```python
from build123d import *

# Parameters (mm, degrees)
SALIENTE_EXTRUIR1_DEPTH = 12.7
CORTAR_EXTRUIR20_DEPTH  = 62
CROQUIS12_R             = 26
CROQUIS12_R_2           = 17
CORTAR_EXTRUIR21_DEPTH  = 4
CROQUIS6_R              = 1.25
CORTAR_EXTRUIR22_DEPTH  = 29
CROQUIS13_R             = 1.5
CORTAR_EXTRUIR23_DEPTH  = 29
CROQUIS8_R              = 3
CORTAR_EXTRUIR27_DEPTH  = 64
CROQUIS5_R              = 36
CORTAR_EXTRUIR28_DEPTH  = 4
CROQUIS22_R             = 27
CORTAR_EXTRUIR32_DEPTH  = 1
CORTAR_EXTRUIR33_START  = -1
CROQUIS23_R             = 17
CORTAR_EXTRUIR33_DEPTH  = 1
CROQUIS24_R             = 9
CORTAR_EXTRUIR34_DEPTH  = 67


with BuildPart() as part:
    # Croquis2 → Saliente-Extruir1 (new body)
    with BuildSketch(Plane.XY):
        with BuildLine():
            add(Edge.make_bspline(
                [(318.003849686, 21.000507192), (228.612845689, 50.579171404), (93.837740705, 69.713331037), (-40.897656903, 33.469788637), (-68.237071347, 4.559111896)],
                knots=[0, 0, 0, 0, 0.7074371, 1, 1, 1, 1], degree=3))
            Line((-68.237071347, 4.559111896), (-59.653213383, -5.20395025))
            add(Edge.make_bspline(
                [(-31, -25), (-39.39631193, -15.138516418), (-48.385558495, -7.834552383), (-59.653213383, -5.20395025)],
                knots=[0.5325633, 0.5325633, 0.5325633, 0.5325633, 1, 1, 1, 1], degree=3))
            add(Edge.make_bspline(
                [(0, -42), (-18.317933693, -37.788499598), (-31, -25)],
                knots=[0, 0, 0, 0.892929879, 0.892929879, 0.892929879], degree=2))
            add(Edge.make_bspline(
                [(0, -42), (34.804106533, -48.583870116), (140.601557422, -28.662967351), (242.066250638, 5.979270436), (318.003849686, -15.054295763)],
                knots=[0, 0, 0, 0, 0.322299538, 1, 1, 1, 1], degree=3))
            ThreePointArc((318.003849686, -15.054295763), (319.540823222, -15.003980459), (321.071215203, -14.853250005))
            ThreePointArc((321.071215203, -14.853250005), (322.775428516, -14.025460634), (323.64375194, -12.341538815))
            add(Edge.make_bspline(
                [(338, 6.2), (337.96483394, 6.165565228), (334.391730923, 4.926696382), (325.456575586, -0.138969503), (325.231234185, -2.170240746), (323.64375194, -12.341538815)],
                knots=[0.205943753, 0.205943753, 0.205943753, 0.205943753, 0.210383616, 0.534400108, 0.959977028, 0.959977028, 0.959977028, 0.959977028], degree=3))
            ThreePointArc((338, 6.2), (339.38638351, 10.840617369), (336.189590247, 14.479010095))
            Line((336.189590247, 14.479010095), (318.003849686, 21.000507192))
        make_face()
    extrude(amount=SALIENTE_EXTRUIR1_DEPTH)

    # Croquis15 → Cortar-Extruir20 (cut)
    with BuildSketch(Plane.XY.offset(12.7)):
        with BuildLine():
            Line((97.723501447, -12.756776492), (105.361190757, 30.558712033))
            ThreePointArc((105.361190757, 30.558712033), (107.138627567, 33.576200952), (110.459727005, 34.68742528))
            Line((110.459727005, 34.68742528), (185.414039032, 32.069963027))
            ThreePointArc((185.414039032, 32.069963027), (190.128162759, 28.12247669), (187.449594034, 22.587959504))
            Line((187.449594034, 22.587959504), (104.857592698, -18.110066768))
            ThreePointArc((104.857592698, -18.110066768), (99.646563775, -17.624284866), (97.723501447, -12.756776492))
        make_face()
        with BuildLine():
            Line((89.822655638, -11.494535825), (96.768582744, 27.897774295))
            ThreePointArc((96.768582744, 27.897774295), (95.058482028, 32.596237399), (90.134443263, 33.464478287))
            Line((90.134443263, 33.464478287), (52.546738431, 19.783672554))
            ThreePointArc((52.546738431, 19.783672554), (49.332800383, 15.953450339), (51.0429011, 11.254987235))
            Line((51.0429011, 11.254987235), (81.684678824, -14.456517153))
            ThreePointArc((81.684678824, -14.456517153), (86.608717589, -15.324758041), (89.822655638, -11.494535825))
        make_face()
        with BuildLine():
            Line((178.485600868, 8.76169092), (208.786453861, 25.718640542))
            ThreePointArc((208.786453861, 25.718640542), (210.340015249, 26.275882173), (211.990356529, 26.296974372))
            Line((211.990356529, 26.296974372), (242.009853595, 21.667000055))
            ThreePointArc((242.009853595, 21.667000055), (246.246230456, 16.846807749), (242.248805987, 11.826674245))
            Line((242.248805987, 11.826674245), (181.928455927, -0.50030106))
            ThreePointArc((181.928455927, -0.50030106), (176.240671419, 2.65632611), (178.485600868, 8.76169092))
        make_face()
    extrude(amount=-CORTAR_EXTRUIR20_DEPTH, mode=Mode.SUBTRACT)

    # Croquis12 → Cortar-Extruir21 (cut)
    with BuildSketch(Plane(origin=(0, 0, 0), x_dir=(-1, 0, 0), z_dir=(0, 0, -1))):
        Circle(CROQUIS12_R)
        Circle(CROQUIS12_R_2, mode=Mode.SUBTRACT)
    extrude(amount=-CORTAR_EXTRUIR21_DEPTH, mode=Mode.SUBTRACT)

    # Croquis6 → Cortar-Extruir22 (cut)
    with BuildSketch(Plane.XY.offset(12.7)):
        with Locations((0, 22)):
            Circle(CROQUIS6_R)
        with Locations((11, 19.052558883)):
            Circle(CROQUIS6_R)
        with Locations((19.052558883, 11)):
            Circle(CROQUIS6_R)
        with Locations((22, 0)):
            Circle(CROQUIS6_R)
        with Locations((19.052558883, -11)):
            Circle(CROQUIS6_R)
        with Locations((11, -19.052558883)):
            Circle(CROQUIS6_R)
        with Locations((0, -22)):
            Circle(CROQUIS6_R)
        with Locations((-11, -19.052558883)):
            Circle(CROQUIS6_R)
        with Locations((-19.052558883, -11)):
            Circle(CROQUIS6_R)
        with Locations((-22, 0)):
            Circle(CROQUIS6_R)
        with Locations((-19.052558883, 11)):
            Circle(CROQUIS6_R)
        with Locations((-11, 19.052558883)):
            Circle(CROQUIS6_R)
    extrude(amount=-CORTAR_EXTRUIR22_DEPTH, mode=Mode.SUBTRACT)

    # Croquis13 → Cortar-Extruir23 (cut)
    with BuildSketch(Plane(origin=(0, 0, 0), x_dir=(-1, 0, 0), z_dir=(0, 0, -1))):
        with Locations((12.557035742, -3.364647586)):
            Circle(CROQUIS13_R)
        with Locations((3.364647586, -12.557035742)):
            Circle(CROQUIS13_R)
        with Locations((-9.192388155, -9.192388155)):
            Circle(CROQUIS13_R)
        with Locations((9.192388155, 9.192388155)):
            Circle(CROQUIS13_R)
        with Locations((-12.557035742, 3.364647586)):
            Circle(CROQUIS13_R)
        with Locations((-3.364647586, 12.557035742)):
            Circle(CROQUIS13_R)
    extrude(amount=-CORTAR_EXTRUIR23_DEPTH, mode=Mode.SUBTRACT)

    # Croquis8 → Cortar-Extruir27 (cut)
    with BuildSketch(Plane.XY.offset(12.7)):
        with Locations((319.95126245, 5.58477006)):
            Circle(CROQUIS8_R)
    extrude(amount=-CORTAR_EXTRUIR27_DEPTH, mode=Mode.SUBTRACT)

    # Croquis5 → Cortar-Extruir28 (cut)
    with BuildSketch(Plane.XY.offset(12.7)):
        Circle(CROQUIS5_R)
    extrude(amount=-CORTAR_EXTRUIR28_DEPTH, mode=Mode.SUBTRACT)

    # Croquis22 → Cortar-Extruir32 (cut)
    with BuildSketch(Plane.XY.offset(8.7)):
        Circle(CROQUIS22_R)
    extrude(amount=-CORTAR_EXTRUIR32_DEPTH, mode=Mode.SUBTRACT)

    # Croquis23 → Cortar-Extruir33 (cut)
    with BuildSketch(Plane.XY.offset(7.7).offset(CORTAR_EXTRUIR33_START)):
        with Locations(Location((0, 0, 0), (0, 0, 180))):
            Circle(CROQUIS23_R)
    extrude(amount=CORTAR_EXTRUIR33_DEPTH, mode=Mode.SUBTRACT)

    # Croquis24 → Cortar-Extruir34 (cut)
    with BuildSketch(Plane(origin=(0, 0, 0), x_dir=(-1, 0, 0), z_dir=(0, 0, -1))):
        Circle(CROQUIS24_R)
    extrude(amount=-CORTAR_EXTRUIR34_DEPTH, mode=Mode.SUBTRACT)


solid = part.part
```
Check sheet for the modelled part. Datum: model origin and axes. Units: mm. A direction names the side the tool comes from. Coordinates: 2 decimals unless noted, no trailing zeros. Answer as a JSON object with one key per item and string values.
1. Depth check by flat-ended pin: P1, Ø1.5, axis at x = -19.05, y = 11, coming from the +Z side; P2, Ø6, axis at y = 0.5, z = 2.5, coming from the -X side; P3, Ø3, axis at x = -11, y = -19.05, coming from the -Z side; P4, Ø21.5, axis at x = -2.5, y = 6, coming from the +Z side. Enter the tip coordinate at first touch or a pass-through.
Outcome:
{"P1": "through", "P2": "x = -67.31", "P3": "z = 4", "P4": "z = 7.7"}
2. Access from +Z, -Z, +X, -X, +Y, -Y to the whole of each face (thin tool, end or side, straight path). Record for faces 3 (the flat face through (66.15, -1.42, 6.44)), 4 (the cylindrical face through (20.633, -15.821, 1.972)), 5 (the flat face through (18, 0, 7.7)).
Outcome:
{"face 3": "+Z, -Z", "face 4": "-Z", "face 5": "+Z"}
3. Release check for a two-part mould opening along Y. For faces 1 (the flat face through (7, -7, 0)), 2 (the cylindrical face through (190.11, 28.21, 6.44)) record: pulls with the +Y half, pulls with the -Y half, needs draft (parallel to the pull), parting line crosses it, or undercut.
Outcome:
{"face 1": "needs draft", "face 2": "undercut"}
4. Scan lines: L1, parallel to Y at x = 11, z = 5.35; L2, parallel to Y at x = 0, z = 1.75; L3, parallel to Y at x = 0, z = 7.45. Record each from-to range of solid material in increasing order. Write a range as from..to.
Outcome:
{"L1": "-43.66..-20.3, -17.8..17.8, 20.3..45", "L2": "-42..-26, -17..-9, 9..17, 26..42.27", "L3": "-42..-23.25, -20.75..-17, 17..20.75, 23.25..42.27"}
